Build history of the part. All positions in model axes, mm. Give positions to 0.01 mm unless a question says otherwise; leave off trailing zeros. Order: outer loops, then holes, each group sorted by start corner. A loop starts at its lowest first (then second) coordinate and runs counter-clockwise, first axis right, second up. Notation, with made-up numbers: (89.5, 31) - (142.5, 31) arc R9 cw to (142.5, 43) - close; hole circle Ø3 at (22, 74). An arc over 180 degrees is marked (long way). Use a Markdown table: item, result. Add a question column.
(1) Wall check: line 1 (Y direction, x = 43.5, z = 2.2); line 2 (X direction, y = -2, z = 0.8); line 3 (X direction, y = -1.5, z = 0.1). Give the ranges that are in metal, low to high.
(2) Slice it at A-A (x = -22.5). Write the cut outline in (y, z), then the cut area to 3 significant figures.
(3) Slice it at C-C (z = 0.5). Write the cut outline in (x, y).
(4) Slice it at B-B (y = 0). Write the cut outline in (x, z), then the cut area to 3 significant figures.
(5) Flat gauge pin, fed straight in: pin 1 (9 mm diameter, centred on x = -20.96, y = 9.31, fed in from -Z). Where does the tip first touch, or does it go through?
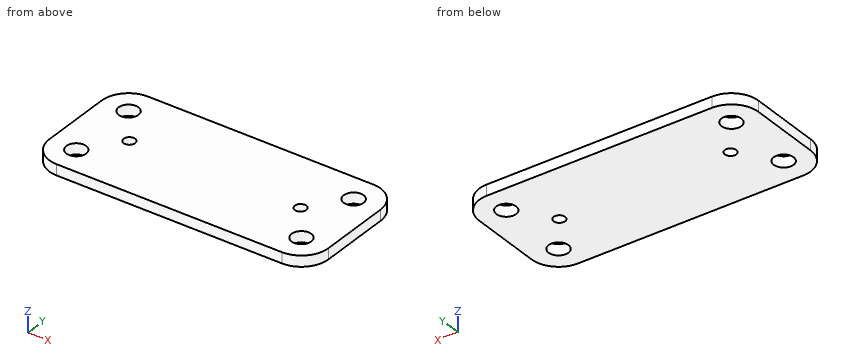
from build123d import *

# Parameters (mm, degrees)
F1_DEPTH = 3
F2_D     = 5.5
F3_D     = 3.2


with BuildPart() as f1:
    # F0 (on Top) → F1 (new body)
    with BuildSketch(Plane.XY):
        with BuildLine():
            Line((41.6422729686, 16.8069582433), (-20.9577269852, 16.8069582433))
            ThreePointArc((-20.9577269852, 16.8069582433), (-15.6544261263, 14.6102591021), (-13.4577269852, 9.3069582433))
            ThreePointArc((-13.4577269852, 9.3069582433), (-20.9577269852, 1.8069582433), (-28.4577269852, 9.3069582433))
            Line((-28.4577269852, 9.3069582433), (-28.4577269852, -10.6930417567))
            ThreePointArc((-28.4577269852, -10.6930417567), (-20.9577269852, -3.1930417567), (-13.4577269852, -10.6930417567))
            ThreePointArc((-13.4577269852, -10.6930417567), (-15.6544261263, -15.9963426156), (-20.9577269852, -18.1930417567))
            Line((-20.9577269852, -18.1930417567), (41.6422730148, -18.1930417567))
            ThreePointArc((41.6422730148, -18.1930417567), (36.3389721559, -5.3897408979), (49.1422730148, -10.6930417567))
            Line((49.1422730148, -10.6930417567), (49.1422730148, 9.3069582433))
            ThreePointArc((49.1422730148, 9.3069582433), (36.3389721722, 4.003657368), (41.6422729686, 16.8069582433))
        make_face()
        with BuildLine():
            ThreePointArc((49.1422730148, 9.3069582433), (46.9455738573, 14.6102591185), (41.6422729686, 16.8069582433))
            ThreePointArc((41.6422729686, 16.8069582433), (36.3389721722, 4.003657368), (49.1422730148, 9.3069582433))
        make_face()
        with BuildLine():
            ThreePointArc((-13.4577269852, 9.3069582433), (-15.6544261263, 14.6102591021), (-20.9577269852, 16.8069582433))
            ThreePointArc((-20.9577269852, 16.8069582433), (-26.2610278441, 14.6102591022), (-28.4577269852, 9.3069582433))
            ThreePointArc((-28.4577269852, 9.3069582433), (-20.9577269852, 1.8069582433), (-13.4577269852, 9.3069582433))
        make_face()
        with BuildLine():
            ThreePointArc((-13.4577269852, -10.6930417567), (-20.9577269852, -3.1930417567), (-28.4577269852, -10.6930417567))
            ThreePointArc((-28.4577269852, -10.6930417567), (-26.2610278441, -15.9963426156), (-20.9577269852, -18.1930417567))
            ThreePointArc((-20.9577269852, -18.1930417567), (-15.6544261263, -15.9963426156), (-13.4577269852, -10.6930417567))
        make_face()
        with BuildLine():
            ThreePointArc((41.6422730148, -18.1930417567), (46.9455738737, -15.9963426156), (49.1422730148, -10.6930417567))
            ThreePointArc((49.1422730148, -10.6930417567), (36.3389721559, -5.3897408979), (41.6422730148, -18.1930417567))
        make_face()
    extrude(amount=F1_DEPTH)

    # F2 (through all)
    with Locations(Plane(origin=(0, 0, 0), x_dir=(1, 0, 0), z_dir=(0, 0, -1))):
        with Locations((-20.9577269852, -9.3069582433), (-20.9577269852, 10.6930417567), (41.6422730148, 10.6930417567), (41.6422730148, -9.3069582433)):
            Hole(F2_D / 2)

    # F3 (through all)
    with Locations(Plane(origin=(0, 0, 0), x_dir=(1, 0, 0), z_dir=(0, 0, -1))):
        with Locations((-13.4577269852, 0.6930417567), (34.1422730148, 0.6930417567)):
            Hole(F3_D / 2)


solid = f1.part
Solution:
| question | item | result |
|---|---|---|
| 1 | line 1 | -17.96 to -12.72, -8.67 to 7.28, 11.33 to 16.57 |
| 1 | line 2 | -28.46 to -14.38, -12.53 to 33.22, 35.07 to 49.14 |
| 1 | line 3 | -28.46 to -14.84, -12.08 to 32.76, 35.52 to 49.14 |
| 2 | outline | (-18.03, 0) - (-12.97, 0) - (-12.97, 3) - (-18.03, 3) - close; (-8.42, 0) - (7.03, 0) - (7.03, 3) - (-8.42, 3) - close; (11.58, 0) - (16.65, 0) - (16.65, 3) - (11.58, 3) - close |
| 2 | area | 76.7 mm2 |
| 3 | outline | (-28.46, -10.69) arc R7.5 ccw to (-20.96, -18.19) - (41.64, -18.19) arc R7.5 ccw to (49.14, -10.69) - (49.14, 9.31) arc R7.5 ccw to (41.64, 16.81) - (-20.96, 16.81) arc R7.5 ccw to (-28.46, 9.31) - close; hole circle Ø5.5 at (-20.96, -10.69); hole circle Ø5.5 at (-20.96, 9.31); hole circle Ø3.2 at (-13.46, -0.69); hole circle Ø3.2 at (34.14, -0.69); hole circle Ø5.5 at (41.64, -10.69); hole circle Ø5.5 at (41.64, 9.31) |
| 4 | outline | (-28.46, 0) - (-14.9, 0) - (-14.9, 3) - (-28.46, 3) - close; (-12.02, 0) - (32.7, 0) - (32.7, 3) - (-12.02, 3) - close; (35.58, 0) - (49.14, 0) - (49.14, 3) - (35.58, 3) - close |
| 4 | area | 215 mm2 |
| 5 | pin 1 | z = 0 |
